Part model, mm, in its own coordinate system. Face numbers are marked on the shaded views. Give positions to 0.01 mm unless a question says otherwise; leave off trailing zeros. Write each loop counter-clockwise with the first axis right and the second up, starting at its lowest first coordinate (ties: lowest second). Pieces come first, ordered by that corner, then holes. Notation, with made-up numbers: M 10.5,70 L 54.5,70 A24 ccw 54.5,96 Z; hole C -39,20.25 d10. An arc over 180 degrees is marked long. Use a Markdown table: item, result.
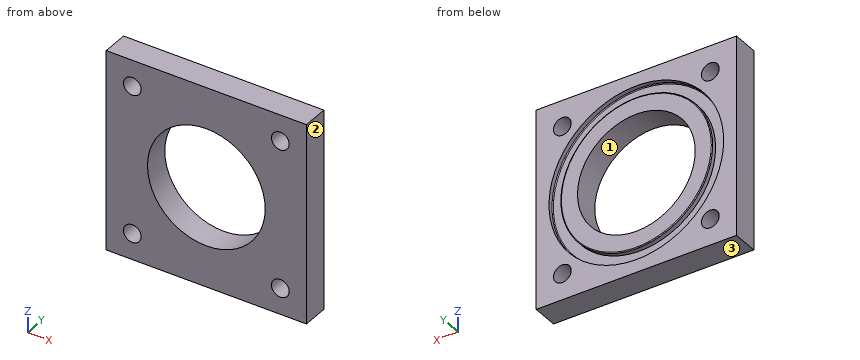
```python
from build123d import *

# Parameters (mm, degrees)
F0_W      = 48.6210244843
F0_H      = 48.6210244843
F0_R      = 2.15265
F1_DEPTH  = 6.35
F6_W      = 2.794
F6_H      = 1.27
F8_R      = 0.2032
F9_R      = 14.2875
F10_DEPTH = 6.351


with BuildPart() as f1:
    # F0 (on Front) → F1 (new body)
    with BuildSketch(Plane.XZ):
        Rectangle(F0_W, F0_H)
        with Locations((-17.9605122421, -17.9605122421)):
            Circle(F0_R, mode=Mode.SUBTRACT)
        with Locations((17.9605122421, -17.9605122421)):
            Circle(F0_R, mode=Mode.SUBTRACT)
        with Locations((-17.9605122421, 17.9605122421)):
            Circle(F0_R, mode=Mode.SUBTRACT)
        with Locations((17.9605122421, 17.9605122421)):
            Circle(F0_R, mode=Mode.SUBTRACT)
    extrude(amount=F1_DEPTH)

    # F6 (on 3pt) → F7 (revolve, cut)
    with BuildSketch(Plane(origin=(0, 0, 0), x_dir=(1, 0, 0), z_dir=(0, 0, -1))):
        with Locations((-19.7993, 0.635)):
            Rectangle(F6_W, F6_H)
    revolve(axis=Axis((0, 0.4501026124, 0), (0, -1, 0)), mode=Mode.SUBTRACT)

    # F8
    f8_edges = [f1.edges().sort_by_distance(p)[0] for p in [
        (21.1963, -1.27, 0),
        (18.4023, 0, 0),
    ]]
    fillet(f8_edges, radius=F8_R)

    # F9 (on face) → F10 (cut, through all)
    with BuildSketch(Plane(origin=(0, 0, 0), x_dir=(-1, 0, 0), z_dir=(0, 1, 0))):
        Circle(F9_R)
    extrude(amount=-F10_DEPTH, mode=Mode.SUBTRACT)


solid = f1.part
```
1. Cut at C-C, the plane y = -4. Give the cut face in (x, z) (1 decimal).
Findings below:
| item | result |
|---|---|
| outline | M -24.3,-24.3 L 24.3,-24.3 L 24.3,24.3 L -24.3,24.3 Z; hole C -18,-18 d4.3; hole C -18,18 d4.3; hole C 0,0 d28.6; hole C 18,-18 d4.3; hole C 18,18 d4.3 |
2. Cut at B-B, the plane x = 0. Give the cut face in (y, z), then the cut area to 3 significant figures.
Findings below:
| item | result |
|---|---|
| outline | M -6.35,-24.31 L 0,-24.31 L 0,-21.2 L -1.07,-21.2 A0.2 cw -1.27,-20.99 L -1.27,-18.4 L -0.2,-18.4 A0.2 ccw 0,-18.2 L 0,-14.29 L -6.35,-14.29 Z; M -6.35,14.29 L 0,14.29 L 0,18.2 A0.2 ccw -0.2,18.4 L -1.27,18.4 L -1.27,20.99 A0.2 cw -1.07,21.2 L 0,21.2 L 0,24.31 L -6.35,24.31 Z |
| area | 120 mm2 |
3. Cut at A-A, the plane z = 0. Give the cut face in (x, y).
Findings below:
| item | result |
|---|---|
| outline | M -24.31,-6.35 L -14.29,-6.35 L -14.29,0 L -18.2,0 A0.2 ccw -18.4,-0.2 L -18.4,-1.27 L -20.99,-1.27 A0.2 cw -21.2,-1.07 L -21.2,0 L -24.31,0 Z; M 14.29,-6.35 L 24.31,-6.35 L 24.31,0 L 21.2,0 L 21.2,-1.07 A0.2 cw 20.99,-1.27 L 18.4,-1.27 L 18.4,-0.2 A0.2 ccw 18.2,0 L 14.29,0 Z |
4. Two-plate mould, pull along X, no slides. Class the marked faces 1, 2 and 3: released by +X, released by -X, zero draft, split by the parting line, or undercut.
Findings below:
| item | result |
|---|---|
| face 1 | undercut |
| face 2 | released by +X |
| face 3 | zero draft |
5. Cut at D-D, the plane z = -19.5. State how many separate pieces and enclosed holes the cut face has, then the cut area to 3 significant figures.
Findings below:
| item | result |
|---|---|
| separate pieces | 3 |
| enclosed holes | 0 |
| area | 249 mm2 |
6. Drill centre lines: L1, parallel to Z at x = -19.5, y = -3; L2, parallel to Z at x = -19, y = -3.5; L3, parallel to Z at x = 0, y = -2.75. Where is each one in solid material? Low to high.
Findings below:
| item | result |
|---|---|
| L1 | -24.31 to -19.47, -16.46 to 16.46, 19.47 to 24.31 |
| L2 | -24.31 to -19.85, -16.08 to 16.08, 19.85 to 24.31 |
| L3 | -24.31 to -14.29, 14.29 to 24.31 |
